Part model, mm, in its own coordinate system. A direction names the side the tool comes from. Coordinates: 2 decimals unless noted, no trailing zeros. Order: outer loops, then holes, each group sorted by start corner. A loop starts at its lowest first (then second) coordinate and runs counter-clockwise, first axis right, second up. Notation, with made-up numbers: M 23,72.5 L 73,72.5 A9 ccw 73,86.5 Z; hole C -13,45 d6. An arc over 180 degrees is marked long. Answer in a Markdown table with one row per item. Add a question column.
from build123d import *

# Parameters (mm, degrees)
F0_R     = 4.445
F1_DEPTH = 3.175
F0_R_2   = 5.715
F2_DEPTH = 0.635
F3_START = -0.635
F0_R_3   = 9.525
F3_DEPTH = 1.905


with BuildPart() as f1:
    # F0 (on Top) → F1 (new body)
    with BuildSketch(Plane.XY):
        Circle(F0_R)
    extrude(amount=F1_DEPTH)

    # F0 (on Top) → F2 (join)
    with BuildSketch(Plane.XY):
        Circle(F0_R_2)
        Circle(F0_R, mode=Mode.SUBTRACT)
        Circle(F0_R)
    extrude(amount=-F2_DEPTH)

    # F0 (on Top) → F3 (join)
    with BuildSketch(Plane.XY.offset(F3_START)):
        Circle(F0_R_3)
        Circle(F0_R_2, mode=Mode.SUBTRACT)
        Circle(F0_R_2)
        Circle(F0_R, mode=Mode.SUBTRACT)
        Circle(F0_R)
    extrude(amount=-F3_DEPTH)


solid = f1.part
(1) Drop a flat-ended pin along its axis: P1, Ø6, axis at x = 4, y = 4, coming from the +Z side (3 decimals). Give the stop position or say it passes through.
(2) Wall check: line 1 (Z direction, x = 8, y = -1.5) (3 decimals); line 2 (Z direction, x = 1.5, y = -5.25); line 3 (Y direction, x = 6.5, z = -1.3). Give the ranges that are in metal, low to high.
(3) Slice it at D-D (y = 4.75). List the corners of the cut face in (x, z) (3 decimals), and give its area (3 significant figures).
(4) Slice it at A-A (y = 0). List the corners of the cut face in (x, z) (3 decimals), and give its area (3 significant figures).
(5) Pull direction Y, two halves, no side cores. Call faces 3 (the cylindrical face through (-0.96, -4.34, 1.57)), 4 (the flat face through (0, 0, -2.54)): pulls with the +Y half, pulls with the -Y half, needs draft (parallel to the pull), parting line crosses it, or undercut.
(6) 3-axis set-ups, long thin cutter, end or side, ignore diameter. For faces 1 (the flat face through (0, -5, 0)), 2 (the flat face through (0, 0, 3.175)): which of +Z, -Z, +X, -X, +Y, -Y reach the whole face in a straight line?
(7) Slice it at C-C (z = 2.8). List the corners of the cut face in (x, y) (3 decimals).
Computed:
| question | item | result |
|---|---|---|
| 1 | P1 | stops at z = 3.175 |
| 2 | line 1 | z = -2.54 to -0.635 |
| 2 | line 2 | z = -2.54 to 0 |
| 2 | line 3 | y = -6.96 to 6.96 |
| 3 | outline | M -8.256,-2.54 L 8.256,-2.54 L 8.256,-0.635 L 3.178,-0.635 L 3.178,0 L -3.178,0 L -3.178,-0.635 L -8.256,-0.635 Z |
| 3 | area | 35.5 mm^2 |
| 4 | outline | M -9.525,-2.54 L 9.525,-2.54 L 9.525,-0.635 L 5.715,-0.635 L 5.715,0 L 4.445,0 L 4.445,3.175 L -4.445,3.175 L -4.445,0 L -5.715,0 L -5.715,-0.635 L -9.525,-0.635 Z |
| 4 | area | 71.8 mm^2 |
| 5 | face 3 | parting line crosses it |
| 5 | face 4 | needs draft |
| 6 | face 1 | +Z |
| 6 | face 2 | +Z, +X, -X, +Y, -Y |
| 7 | outline | C 0,0 d8.89 |
